Autodesk Inventor part; units mm, degrees
ref_plane "YZ Plane" through (0, 0, 0) normal (1, 0, 0) x (0, 1, 0)
ref_plane "XZ Plane" through (0, 0, 0) normal (0, 1, 0) x (-1, 0, 0)
ref_plane "XY Plane" through (0, 0, 0) normal (0, 0, 1) x (1, 0, 0)
sketch "Sketch1" plane through (0, 0, 0) normal (0, 1, 0) x (-1, 0, 0)
  circle A0 centre (0, 0) radius 20
  dimension "d24" = 40
extrude "Extrusion1" add sketch "Sketch1" along normal blind 50
sketch "Sketch2" plane through (0, 50, 0) normal (0, 1, 0) x (1, 0, 0)
  circle A0 centre (0, 0) radius 55
  dimension "d3" = 110
extrude "Extrusion2" add sketch "Sketch2" against normal blind 50
sketch "Sketch3" plane through (0, 50, 0) normal (0, 1, 0) x (1, 0, 0)
  circle A0 centre (0, 0) radius 5
  dimension "d6" = 10
extrude "Extrusion3" cut sketch "Sketch3" against normal blind 50
sketch "Sketch4" plane through (0, 50, 0) normal (0, 1, 0) x (1, 0, 0)
  circle A0 centre (0, -45) radius 5
  point P0 (0, 0)
  dimension "d9" = 10
extrude "Extrusion4" add sketch "Sketch4" along normal blind 1
sketch "Sketch5" plane through (0, 50, 0) normal (0, 1, 0) x (1, 0, 0)
  circle A0 centre (0, 0) radius 40
  dimension "d12" = 80
extrude "Extrusion5" cut sketch "Sketch5" against normal through all keep common part
sketch "Sketch6" plane through (0, 50, 0) normal (0, 1, 0) x (1, 0, 0)
  circle A0 centre (0, 0) radius 40
sketch "Sketch7" plane through (0, 0, 0) normal (0, -1, 0) x (1, 0, 0)
  circle A0 centre (0, 0) radius 40
extrude "Extrusion6" cut sketch "Sketch7" against normal blind 10
sketch "Sketch8" plane through (0, 50, 0) normal (0, 1, 0) x (1, 0, 0)
  circle A0 centre (0, 30) radius 5
  point P0 (0, 0)
  dimension "d17" = 10
extrude "Extrusion7" add sketch "Sketch8" along normal blind 1
sketch "Sketch9" plane through (0, 50, 0) normal (0, 1, 0) x (1, 0, 0)
  circle A0 centre (0, 0) radius 2.5
  dimension "d20" = 5
sketch "Sketch10" plane through (0, 10, 0) normal (0, -1, 0) x (1, 0, 0)
  circle A0 centre (0, 0) radius 5
  circle A1 centre (0, 0) radius 40
extrude "Extrusion8" cut sketch "Sketch10" against normal blind 10
Input: part model. Units: mm. Frame: model coordinates. Give positions to 0.01 mm unless a question says otherwise; leave off trailing zeros. Order: outer loops, then holes, each group sorted by start corner. A loop starts at its lowest first (then second) coordinate and runs counter-clockwise, first axis right, second up. Notation, with made-up numbers: (-8, -40) - (35, -40) arc R8 ccw to (35, -36) - close; hole circle Ø2 at (11, 79.5). An arc over 180 degrees is marked (long way). Answer as a JSON object with one key per item and string values. Group by question number.
Q1. Cut plane C-C, the plane y = 40.5. Output: boundary loops of the cut face in (x, z), then the cut area to 3 significant figures.
Q2. First-contact query: pin 1 Ø6 at (x, y) = (15.5, 43.5) entering from +Z; pin 2 Ø3 at (x, y) = (4.5, 27) entering from +Z; pin 3 Ø16 at (x, z) = (0, 0) entering from +Y; pin 4 Ø10 at (y, z) = (43.5, 1) entering from -X. Flat tips, straight axial feed; report the tip coordinate or a pass-through.
Q3. Cut plane B-B, the plane x = 0. Output: boundary loops of the cut face in (y, z).
Q4. Mould query, pull axis Z, two halves, no side actions, for faces 1 (the face through (-1.08, 35.21, 4.88)), 2 (the face through (-1, 50, 8)), 3 (the face through (-1.08, 50.49, -34.88)). Classes: pulls with the +Z half, pulls with the -Z half, needs draft (parallel to the pull), parting line crosses it, or undercut.
Q5. Line query: probe 1 along X at (y, z) = (41, 0); probe 2 along Y at (x, z) = (-18.5, -2.5). Output: solid intervals per line, ascending.
Q6. Cut plane D-D, the plane z = -34. Output: boundary loops of the cut face in (x, y).
Q7. Cut plane A-A, the plane z = 0. Output: boundary loops of the cut face in (x, y), then the cut area to 3 significant figures.
Results:
{
 "1": {"outline": "circle Ø80 at (0, 0); hole circle Ø10 at (0, 0)", "area": "4,950 mm^2"},
 "2": {"pin 1": "z = 38", "pin 2": "z = 39.89", "pin 3": "y = 50", "pin 4": "x = -40"},
 "3": {"outline": "(20, -40) - (50, -40) - (50, -35) - (51, -35) - (51, -25) - (50, -25) - (50, -5) - (20, -5) - close; (20, 5) - (50, 5) - (50, 40) - (20, 40) - close"},
 "4": {"face 1": "undercut", "face 2": "needs draft", "face 3": "parting line crosses it"},
 "5": {"probe 1": "-40 to -5, 5 to 40", "probe 2": "20 to 50"},
 "6": {"outline": "(-21.07, 20) - (21.07, 20) - (21.07, 50) - (3, 50) - (3, 51) - (-3, 51) - (-3, 50) - (-21.07, 50) - close"},
 "7": {"outline": "(-40, 20) - (-5, 20) - (-5, 50) - (-40, 50) - close; (5, 20) - (40, 20) - (40, 50) - (5, 50) - close", "area": "2,100 mm^2"}
}
